from build123d import *

# Parameters (mm, degrees)
SKETCH1_W                    = 22.5
SKETCH1_H                    = 22.5
BOSS_EXTRUDE1_DEPTH          = 20
CUT_EXTRUDE1_START           = -5
SKETCH3_W                    = 18.5
SKETCH3_H                    = 18.5
CUT_EXTRUDE1_DEPTH           = 12
CUT_EXTRUDE1_TAPER           = 10
CUT_EXTRUDE1_OTHER_WAY_DEPTH = 5
CUT_EXTRUDE2_REACH           = 22
SKETCH2_R                    = 4.375
CUT_EXTRUDE3_REACH           = 24.5
SKETCH4_R                    = 4.25
SKETCH5_W                    = 5
SKETCH5_H                    = 4


with BuildPart() as part:
    # Sketch1 → Boss-Extrude1 (new body)
    with BuildSketch(Plane(origin=(0, 0, 0), x_dir=(1, 0, 0), z_dir=(0, 1, 0))):
        Rectangle(SKETCH1_W, SKETCH1_H)
    extrude(amount=BOSS_EXTRUDE1_DEPTH)

    # Sketch3 → Cut-Extrude1 (cut)
    with BuildSketch(Plane.XZ.offset(CUT_EXTRUDE1_START)):
        Rectangle(SKETCH3_W, SKETCH3_H)
    extrude(amount=-CUT_EXTRUDE1_DEPTH, taper=CUT_EXTRUDE1_TAPER, mode=Mode.SUBTRACT)

    # Sketch3 → Cut-Extrude1 other way (cut)
    with BuildSketch(Plane.XZ.offset(CUT_EXTRUDE1_START)):
        Rectangle(SKETCH3_W, SKETCH3_H)
    extrude(amount=CUT_EXTRUDE1_OTHER_WAY_DEPTH, mode=Mode.SUBTRACT)

    # Sketch2 → Cut-Extrude2 (cut, up to next)
    with BuildSketch(Plane(origin=(0, 20, 0), x_dir=(1, 0, 0), z_dir=(0, 1, 0)), mode=Mode.PRIVATE) as cut_extrude2_sk1:
        Circle(SKETCH2_R)
    cut_extrude2_tool1 = extrude(cut_extrude2_sk1.sketch, amount=-CUT_EXTRUDE2_REACH, mode=Mode.PRIVATE) & part.part
    add(cut_extrude2_tool1.solids().sort_by_distance((0, 20, 0))[0], mode=Mode.SUBTRACT)

    # Sketch4 → Cut-Extrude3 (cut, up to next)
    with BuildSketch(Plane(origin=(11.25, 0, 0), x_dir=(0, 0, -1), z_dir=(1, 0, 0)), mode=Mode.PRIVATE) as cut_extrude3_sk1:
        with Locations((0, 10)):
            Circle(SKETCH4_R)
    cut_extrude3_tool1 = extrude(cut_extrude3_sk1.sketch, amount=-CUT_EXTRUDE3_REACH, mode=Mode.PRIVATE) & part.part
    add(cut_extrude3_tool1.solids().sort_by_distance((11.25, 10, 0))[0], mode=Mode.SUBTRACT)

    # Sweep1: sweep along a path in Sketch6
    with BuildLine(Plane(origin=(0, 0, 0), x_dir=(0, 0, -1), z_dir=(1, 0, 0))) as sweep1_path:
        Line((11.25, 10), (14.25, 10))
        ThreePointArc((14.25, 10), (15.912838742, 10.235022349), (17.445409396, 10.921677561))
    # Sketch5 → Sweep1 (sweep)
    with BuildSketch(Plane(origin=(0, 0, -11.25), x_dir=(-1, 0, 0), z_dir=(0, 0, -1))):
        with Locations((0, 10)):
            Rectangle(SKETCH5_W, SKETCH5_H)
    sweep1 = sweep(path=sweep1_path.line)

    # Mirror1: Sweep1 across plane
    add(sweep1.mirror(Plane.XY))


solid = part.part
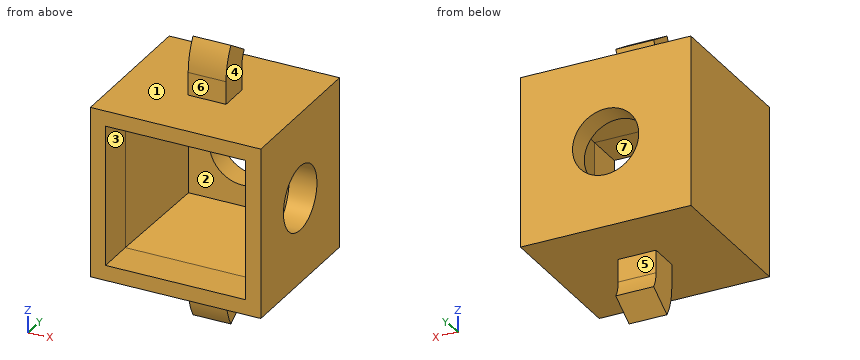
The model under review builds one solid part; all positions refer to its coordinate system, in mm. Face numbers are marked on the shaded views. A direction names the side the tool comes from. Coordinates: 2 decimals unless noted, no trailing zeros. Write each loop counter-clockwise with the first axis right and the second up, starting at its lowest first coordinate (ties: lowest second). Pieces come first, ordered by that corner, then holes. Notation, with made-up numbers: (-33, -11) -> (-23, -11) arc R32 ccw to (-23, 20) -> close; hole circle Ø10 at (-25, -30.5). An arc over 180 degrees is marked (long way). Answer in a Markdown table with one row per item.
1. We need section D-D, the plane y = 18.5. State the section outline as (x, z) points (3 decimals).
Answers below:
| item | result |
|---|---|
| outline | (-11.25, -11.25) -> (11.25, -11.25) -> (11.25, 11.25) -> (-11.25, 11.25) -> close; hole circle Ø8.75 at (0, 0) |
2. Draft analysis for pull direction X (two halves, no side actions). For the marked faces 1, 2, 3 and 4, state which applies: +X half, -X half, draft (parallel to the pull), parting line (faces both ways), or undercut.
Answers below:
| item | result |
|---|---|
| face 1 | draft |
| face 2 | undercut |
| face 3 | undercut |
| face 4 | +X half |
3. We need section A-A, the plane y = 1.5. State the section outline as (x, z) points.
Answers below:
| item | result |
|---|---|
| outline | (-11.25, -11.25) -> (11.25, -11.25) -> (11.25, 11.25) -> (-11.25, 11.25) -> close; hole (-9.25, -9.25) -> (9.25, -9.25) -> (9.25, 9.25) -> (-9.25, 9.25) -> close |
4. Wall thickness on probe 1 along X at (y, z) = (19.45, 0) (3 decimals); probe 2 along Z at (x, y) = (5, 4): over which ranges is each line inside the solid? List them lowest first. Write a range as [from, to].
Answers below:
| item | result |
|---|---|
| probe 1 | x = [-11.25, -4.375], [4.375, 11.25] |
| probe 2 | z = [-11.25, -9.25], [9.25, 11.25] |
5. We need section C-C, the plane z = -13.5. State the section outline as (x, y) points, and give its area (3 significant figures).
Answers below:
| item | result |
|---|---|
| outline | (-2.5, 8) -> (2.5, 8) -> (2.5, 12) -> (-2.5, 12) -> close |
| area | 20.0 mm^2 |
6. Clearance check with flat-ended pins moving along their axes: pin 1 Ø1.5 at (x, y) = (2.5, 3.5) entering from +Z; pin 2 Ø0.9 at (x, z) = (-1, 13) entering from +Y; pin 3 Ø5 at (y, z) = (9.5, -16) entering from +X. State where each tip first meets the part, or that it passes through.
Answers below:
| item | result |
|---|---|
| pin 1 | stops at z = 11.25 |
| pin 2 | stops at y = 12 |
| pin 3 | stops at x = 2.5 |
7. For the marked faces 5, 6 and 7, list the 3-axis set-ups (+Z, -Z, +X, -X, +Y, -Y) from which the entire face can be reached by the end or side of a thin tool; tool diameter is ignored.
Answers below:
| item | result |
|---|---|
| face 5 | +X, -X, +Y |
| face 6 | +Z, +X, -X, -Y |
| face 7 | -Y |
8. We need section B-B, the plane x = 9.75. State the section outline as (y, z) points, and give its area (3 significant figures).
Answers below:
| item | result |
|---|---|
| outline | (0, -11.25) -> (20, -11.25) -> (20, 11.25) -> (0, 11.25) -> close; hole circle Ø8.5 at (10, 0) |
| area | 393 mm^2 |
